Could you check a few things on this model? Use its own coordinates, in mm. A direction names the side the tool comes from. Give positions to 0.01 mm unless a question says otherwise; leave off trailing zeros. Write each loop counter-clockwise with the first axis right and the second up, starting at its lowest first coordinate (ties: lowest second). Pieces come first, ordered by that corner, then holes. Notation, with made-up numbers: (-38.75, 9.5) - (-1.75, 9.5) arc R23 ccw to (-1.75, 26.5) - close; hole circle Ø1 at (-19, 51.25). An arc over 180 degrees is marked (long way). Use one line per item in the form item = value.
```python
from build123d import *

# Parameters (mm, degrees)
SKETCH1_W           = 254
SKETCH1_H           = 177.8
BOSS_EXTRUDE1_DEPTH = 101.6
SKETCH4_R           = 12.7
CUT_EXTRUDE3_DEPTH  = 50.8
SKETCH6_R           = 12.7
CUT_EXTRUDE4_DEPTH  = 50.8
SKETCH7_R           = 12.7
CUT_EXTRUDE5_DEPTH  = 33.02


with BuildPart() as part:
    # Sketch1 → Boss-Extrude1 (new body)
    with BuildSketch(Plane.XY):
        Rectangle(SKETCH1_W, SKETCH1_H)
    extrude(amount=BOSS_EXTRUDE1_DEPTH)

    # Sketch4 → Cut-Extrude3 (cut)
    with BuildSketch(Plane.XZ.offset(88.9)):
        with Locations(Location((-101.6, 25.4, 0), (0, 0, 270))):
            Circle(SKETCH4_R)
        with Locations(Location((101.6, 25.4, 0), (0, 0, 270))):
            Circle(SKETCH4_R)
    cut_extrude3 = extrude(amount=-CUT_EXTRUDE3_DEPTH, mode=Mode.SUBTRACT)

    # Mirror4: Cut-Extrude3 across plane
    add(cut_extrude3.mirror(Plane.ZX), mode=Mode.SUBTRACT)

    # Sketch6 → Cut-Extrude4 (cut)
    with BuildSketch(Plane.XZ.offset(88.9)):
        with Locations(Location((0, 76.2, 0), (0, 0, 270))):
            Circle(SKETCH6_R)
    cut_extrude4 = extrude(amount=-CUT_EXTRUDE4_DEPTH, mode=Mode.SUBTRACT)

    # Mirror5: Cut-Extrude4 across plane
    add(cut_extrude4.mirror(Plane.ZX), mode=Mode.SUBTRACT)

    # Sketch7 → Cut-Extrude5 (cut)
    with BuildSketch(Plane.XY.offset(101.6)):
        with Locations((63.5, -50.8)):
            Circle(SKETCH7_R)
        with Locations((63.5, 50.8)):
            Circle(SKETCH7_R)
        with Locations((-63.5, -50.8)):
            Circle(SKETCH7_R)
        with Locations((-63.5, 50.8)):
            Circle(SKETCH7_R)
    extrude(amount=-CUT_EXTRUDE5_DEPTH, mode=Mode.SUBTRACT)


solid = part.part
```
1. Imagine slicing it at B-B, the plane x = 0. List the corners of the cut face in (y, z) for me, and give its area (3 significant figures).
Response values:
outline = (-88.9, 0) - (88.9, 0) - (88.9, 63.5) - (38.1, 63.5) - (38.1, 88.9) - (88.9, 88.9) - (88.9, 101.6) - (-88.9, 101.6) - (-88.9, 88.9) - (-38.1, 88.9) - (-38.1, 63.5) - (-88.9, 63.5) - close
area = 15,500 mm²
2. Which directions (+Z, -Z, +X, -X, +Y, -Y) give clear straight access to the entire face, cutting with the end or side of a thin tool? Please do faces 4 (the face through (-2, 1, 101.6)), 5 (the face through (-2, 88.9, 50)), 6 (the face through (-51.768, 45.936, 85.321)), 7 (the face through (114.192, -63.856, 27.053)), 8 (the face through (0, 38.1, 76)).
Response values:
face_4 = +Z, +X, -X, +Y, -Y
face_5 = +Z, -Z, +X, -X, +Y
face_6 = +Z
face_7 = -Y
face_8 = +Y
3. Imagine slicing it at D-D, the plane y = -70. List the corners of the cut face in (x, z) for me, and give its area (3 significant figures).
Response values:
outline = (-127, 0) - (127, 0) - (127, 101.6) - (-127, 101.6) - close; hole circle Ø25.4 at (-101.6, 25.4); hole circle Ø25.4 at (0, 76.2); hole circle Ø25.4 at (101.6, 25.4)
area = 24,300 mm²
4. Imagine slicing it at A-A, the plane y = -50.8. List the corners of the cut face in (x, z) for me, and give its area (3 significant figures).
Response values:
outline = (-127, 0) - (127, 0) - (127, 101.6) - (76.2, 101.6) - (76.2, 68.58) - (50.8, 68.58) - (50.8, 101.6) - (-50.8, 101.6) - (-50.8, 68.58) - (-76.2, 68.58) - (-76.2, 101.6) - (-127, 101.6) - close; hole circle Ø25.4 at (-101.6, 25.4); hole circle Ø25.4 at (0, 76.2); hole circle Ø25.4 at (101.6, 25.4)
area = 22,600 mm²
5. Imagine slicing it at C-C, the plane z = 25.4. List the corners of the cut face in (x, y) for me.
Response values:
outline = (-127, -88.9) - (-114.3, -88.9) - (-114.3, -38.1) - (-88.9, -38.1) - (-88.9, -88.9) - (88.9, -88.9) - (88.9, -38.1) - (114.3, -38.1) - (114.3, -88.9) - (127, -88.9) - (127, 88.9) - (114.3, 88.9) - (114.3, 38.1) - (88.9, 38.1) - (88.9, 88.9) - (-88.9, 88.9) - (-88.9, 38.1) - (-114.3, 38.1) - (-114.3, 88.9) - (-127, 88.9) - close
6. If we mould it in two halves opening along X, with no side actions, what happens to faces 1 (the face through (-127, -1, 50)), 2 (the face through (-2, -88.9, 50)), 3 (the face through (75.232, -55.664, 85.321))? For each: pulls with the +X half, pulls with the -X half, needs draft (parallel to the pull), parting line crosses it, or undercut.
Response values:
face_1 = pulls with the -X half
face_2 = needs draft
face_3 = undercut
7. If I drill on line 1 (X direction, y = -75, z = 25.4); line 2 (Y direction, x = -63.5, z = 80); line 3 (X direction, y = -70, z = 76), over which ranges is the centre line in solid material (lowest first)? Write a range as from..to.
Response values:
line_1 = -127..-114.3, -88.9..88.9, 114.3..127
line_2 = -88.9..-63.5, -38.1..38.1, 63.5..88.9
line_3 = -127..-12.7, 12.7..127
8. For pin 1 (23 mm diameter, centred on x = -101.6, z = 25.4, fed in from -Y); pin 2 (23 mm diameter, centred on x = -63.5, y = -50.8, fed in from +Z); pin 3 (12.5 mm diameter, centred on x = 100.5, z = 31, fed in from +Y), each with a flat end and sliding along its axis, tell me the tip position at first contact or that it passes through.
Response values:
pin_1 = -38.1
pin_2 = 68.58
pin_3 = 38.1
